Geometry: final body of the model. Coordinates: model frame, mm. A direction names the side the tool comes from. Coordinates: 2 decimals unless noted, no trailing zeros. Write each loop counter-clockwise with the first axis right and the second up, starting at its lowest first coordinate (ties: lowest second). Pieces come first, ordered by that corner, then holes.
from build123d import *

# Parameters (mm, degrees)
BOSS_EXTRUDE1_DEPTH      = 5.46
BOSS_EXTRUDE1_DEPTH_BACK = 4.7
SKETCH1_R                = 1.335
SKETCH2_W                = 6.6
SKETCH2_H                = 1.78
CUT_EXTRUDE1_DEPTH       = 29.274902299
CHAMFER1_SIZE            = 0.4
SKETCH7_R                = 1.5
CUT_EXTRUDE4_DEPTH       = 0.1
CUT_EXTRUDE5_START       = -10.06
SKETCH7_2_R              = 1.5
CUT_EXTRUDE5_DEPTH       = 0.1
SKETCH3_R                = 1.205
CUT_EXTRUDE2_DEPTH       = 2.16
SKETCH4_R                = 1.205
CUT_EXTRUDE3_DEPTH       = 2.16
BOSS_EXTRUDE2_START      = -1.52
BOSS_EXTRUDE2_DEPTH      = 0.5
LPATTERN1_COUNT          = 3
LPATTERN1_PITCH          = 2.54
LPATTERN2_COUNT          = 3
LPATTERN2_PITCH          = 2.54
BOSS_EXTRUDE3_START      = 7.6
BOSS_EXTRUDE3_DEPTH      = 1
BOSS_EXTRUDE4_START      = -8.6
BOSS_EXTRUDE4_DEPTH      = 1


with BuildPart() as part:
    # Sketch1 → Boss-Extrude1 (new, two sides: drawn at the far end of the back side and taken through both)
    with BuildSketch(Plane(origin=(0, 0, 0), x_dir=(1, 0, 0), z_dir=(0, 1, 0)).offset(-BOSS_EXTRUDE1_DEPTH_BACK)):
        Polygon((-13.335, 7.64), (13.335, 7.64), (13.335, 1.74), (7.535, -4.06), (-7.535, -4.06), (-13.335, 1.74), align=None)
        with Locations(Location((10.48, 4.75, 0), (0, 0, 270))):
            Circle(SKETCH1_R, mode=Mode.SUBTRACT)
        with Locations(Location((-10.48, 4.75, 0), (0, 0, 270))):
            Circle(SKETCH1_R, mode=Mode.SUBTRACT)
    extrude(amount=BOSS_EXTRUDE1_DEPTH + BOSS_EXTRUDE1_DEPTH_BACK)

    # Sketch2 → Cut-Extrude1 (cut, through all)
    with BuildSketch(Plane.ZY.offset(13.335)):
        with Locations((0.76, -0.89)):
            Rectangle(SKETCH2_W, SKETCH2_H)
    extrude(amount=-CUT_EXTRUDE1_DEPTH, mode=Mode.SUBTRACT)

    # Chamfer1
    chamfer1_edges = [part.edges().sort_by_distance(p)[0] for p in [
        (0, 0, 4.06),
        (0, -1.78, 4.06),
    ]]
    chamfer(chamfer1_edges, length=CHAMFER1_SIZE)

    # Sketch7 → Cut-Extrude4 (cut)
    # profile 1 of 2: a face of its own
    with BuildSketch(Plane(origin=(0, 5.46, 0), x_dir=(1, 0, 0), z_dir=(0, 1, 0))):
        with Locations(Location((0, 0, 0), (0, 0, 270))):
            Circle(SKETCH7_R)
    # profile 2 of 2: a face of its own
    with BuildSketch(Plane(origin=(0, 5.46, 0), x_dir=(1, 0, 0), z_dir=(0, 1, 0))):
        with BuildLine():
            Line((-1.5, -1.8), (1.5, -1.8))
            ThreePointArc((1.5, -1.8), (2.5, -2.8), (1.5, -3.8))
            Line((1.5, -3.8), (-1.5, -3.8))
            ThreePointArc((-1.5, -3.8), (-2.5, -2.8), (-1.5, -1.8))
        make_face()
        Polygon((-1.5, -2.8), (-0.82259388, -2.12259388), (-0.82259388, -2.482222738), (1.5, -2.482222738), (1.5, -3.117777262), (-0.82259388, -3.117777262), (-0.82259388, -3.47740612), align=None, mode=Mode.SUBTRACT)
    extrude(amount=-CUT_EXTRUDE4_DEPTH, mode=Mode.SUBTRACT)

    # Sketch7<2> → Cut-Extrude5 (cut)
    # profile 1 of 2: a face of its own
    with BuildSketch(Plane(origin=(0, 5.46, 0), x_dir=(1, 0, 0), z_dir=(0, 1, 0)).offset(CUT_EXTRUDE5_START)):
        with Locations(Location((0, 0, 0), (0, 0, 270))):
            Circle(SKETCH7_2_R)
    # profile 2 of 2: a face of its own
    with BuildSketch(Plane(origin=(0, 5.46, 0), x_dir=(1, 0, 0), z_dir=(0, 1, 0)).offset(CUT_EXTRUDE5_START)):
        with BuildLine():
            Line((-1.5, -1.8), (1.5, -1.8))
            ThreePointArc((1.5, -1.8), (2.5, -2.8), (1.5, -3.8))
            Line((1.5, -3.8), (-1.5, -3.8))
            ThreePointArc((-1.5, -3.8), (-2.5, -2.8), (-1.5, -1.8))
        make_face()
        Polygon((-1.5, -2.8), (-0.82259388, -2.12259388), (-0.82259388, -2.482222738), (1.5, -2.482222738), (1.5, -3.117777262), (-0.82259388, -3.117777262), (-0.82259388, -3.47740612), align=None, mode=Mode.SUBTRACT)
    extrude(amount=-CUT_EXTRUDE5_DEPTH, mode=Mode.SUBTRACT)

    # Sketch3 → Cut-Extrude2 (cut)
    with BuildSketch(Plane(origin=(0, 5.46, 0), x_dir=(1, 0, 0), z_dir=(0, 1, 0))):
        with Locations(Location((6.37, 4.75, 0), (0, 0, 270))):
            Circle(SKETCH3_R)
        with BuildLine():
            Line((-6.56, 5.955), (-6.18, 5.955))
            ThreePointArc((-6.18, 5.955), (-4.975, 4.75), (-6.18, 3.545))
            Line((-6.18, 3.545), (-6.56, 3.545))
            ThreePointArc((-6.56, 3.545), (-7.765, 4.75), (-6.56, 5.955))
        make_face()
    extrude(amount=-CUT_EXTRUDE2_DEPTH, mode=Mode.SUBTRACT)

    # Sketch4 → Cut-Extrude3 (cut)
    with BuildSketch(Plane.XZ.offset(4.7)):
        with Locations(Location((8.635, -1.02, 0), (0, 0, 270))):
            Circle(SKETCH4_R)
        with BuildLine():
            Line((-8.825, 0.185), (-8.445, 0.185))
            ThreePointArc((-8.445, 0.185), (-7.24, -1.02), (-8.445, -2.225))
            Line((-8.445, -2.225), (-8.825, -2.225))
            ThreePointArc((-8.825, -2.225), (-10.03, -1.02), (-8.825, 0.185))
        make_face()
    extrude(amount=-CUT_EXTRUDE3_DEPTH, mode=Mode.SUBTRACT)

    # Sketch5 → Boss-Extrude2 (add)
    with BuildSketch(Plane.XZ.offset(4.7).offset(BOSS_EXTRUDE2_START)):
        Polygon((-0.625, -7.64), (-0.625, -9.440000013), (-0.314999987, -9.749999974), (-0.314999987, -16.335000065), (0, -16.65), (0.315000013, -16.335000091), (0.315000013, -9.75), (0.625, -9.440000013), (0.625, -7.64), align=None)
    boss_extrude2 = extrude(amount=-BOSS_EXTRUDE2_DEPTH)

    # LPattern1: Boss-Extrude2 ×3
    with Locations(*[(i * LPATTERN1_PITCH, 0, 0) for i in range(1, LPATTERN1_COUNT)]):
        add(boss_extrude2)

    # LPattern2: Boss-Extrude2 ×3
    with Locations(*[(-i * LPATTERN2_PITCH, 0, 0) for i in range(1, LPATTERN2_COUNT)]):
        add(boss_extrude2)

    # Sketch6 → Boss-Extrude3 (add)
    with BuildSketch(Plane(origin=(0, 0, 0), x_dir=(0, 0, -1), z_dir=(1, 0, 0)).offset(BOSS_EXTRUDE3_START)):
        with BuildLine():
            Line((7.64, -3.18), (12.04, -3.18))
            ThreePointArc((12.04, -3.18), (12.534974747, -2.974974747), (12.74, -2.48))
            Line((12.74, -2.48), (12.74, 3.2))
            ThreePointArc((12.74, 3.2), (12.534974747, 3.694974747), (12.04, 3.9))
            Line((12.04, 3.9), (7.64, 3.9))
            Line((7.64, 3.9), (7.64, 3.4))
            Line((7.64, 3.4), (12.04, 3.4))
            ThreePointArc((12.04, 3.4), (12.181421356, 3.341421356), (12.24, 3.2))
            Line((12.24, 3.2), (12.24, -2.48))
            ThreePointArc((12.24, -2.48), (12.181421356, -2.621421356), (12.04, -2.68))
            Line((12.04, -2.68), (7.64, -2.68))
            Line((7.64, -2.68), (7.64, -3.18))
        make_face()
    extrude(amount=BOSS_EXTRUDE3_DEPTH)

    # Sketch6<2> → Boss-Extrude4 (add)
    with BuildSketch(Plane(origin=(0, 0, 0), x_dir=(0, 0, -1), z_dir=(1, 0, 0)).offset(BOSS_EXTRUDE4_START)):
        with BuildLine():
            Line((7.64, -3.18), (12.04, -3.18))
            ThreePointArc((12.04, -3.18), (12.534974747, -2.974974747), (12.74, -2.48))
            Line((12.74, -2.48), (12.74, 3.2))
            ThreePointArc((12.74, 3.2), (12.534974747, 3.694974747), (12.04, 3.9))
            Line((12.04, 3.9), (7.64, 3.9))
            Line((7.64, 3.9), (7.64, 3.4))
            Line((7.64, 3.4), (12.04, 3.4))
            ThreePointArc((12.04, 3.4), (12.181421356, 3.341421356), (12.24, 3.2))
            Line((12.24, 3.2), (12.24, -2.48))
            ThreePointArc((12.24, -2.48), (12.181421356, -2.621421356), (12.04, -2.68))
            Line((12.04, -2.68), (7.64, -2.68))
            Line((7.64, -2.68), (7.64, -3.18))
        make_face()
    extrude(amount=BOSS_EXTRUDE4_DEPTH)


solid = part.part
Item 1: Set-up query: faces 4 (the flat face through (8, -2.68, -10)), 5 (the flat face through (0, -4.6, 0)), 6 (the cylindrical face through (-7.765, 4.395, -4.724)), 7 (the flat face through (2.5, -3.18, -11.1)), 8 (the flat face through (8.6, 0.4, -12.4)). Return all of +Z, -Z, +X, -X, +Y, -Y with unobstructed straight access to the full face (end or side cutting, diameter ignored); none if empty.
Derived:
face 4: +X, -X
face 5: -Y
face 6: +Y
face 7: -Z, +X, -X, -Y
face 8: -Z, +X, +Y, -Y
Item 2: Section B-B, the plane z = -4.75. Output: boundary loops of the cut face in (x, y) (3 decimals).
Derived:
outline: (-13.335, -4.7) - (-11.815, -4.7) - (-11.815, 5.46) - (-13.335, 5.46) - close; (-9.145, -4.7) - (9.145, -4.7) - (9.145, 5.46) - (7.575, 5.46) - (7.575, 3.3) - (5.165, 3.3) - (5.165, 5.46) - (-4.975, 5.46) - (-4.975, 3.3) - (-7.765, 3.3) - (-7.765, 5.46) - (-9.145, 5.46) - close; (11.815, -4.7) - (13.335, -4.7) - (13.335, 5.46) - (11.815, 5.46) - close
Item 3: Section D-D, the plane z = -1.02. Output: boundary loops of the cut face in (x, y) (3 decimals).
Derived:
outline: (-12.615, -4.7) - (-10.03, -4.7) - (-10.03, -2.54) - (-7.24, -2.54) - (-7.24, -4.7) - (-1.1, -4.7) - (-1.1, -4.6) - (1.1, -4.6) - (1.1, -4.7) - (7.43, -4.7) - (7.43, -2.54) - (9.84, -2.54) - (9.84, -4.7) - (12.615, -4.7) - (12.615, -1.78) - (-12.615, -1.78) - close; (-12.615, 0) - (12.615, 0) - (12.615, 5.46) - (1.1, 5.46) - (1.1, 5.36) - (-1.1, 5.36) - (-1.1, 5.46) - (-12.615, 5.46) - close
Item 4: Material intervals for probe 1 along X at (y, z) = (3, -4.75) (3 decimals); probe 2 along X at (y, z) = (-3.65, -1.02) (3 decimals); probe 3 along Y at (x, z) = (-2.25, -1.25), sorted ascending.
Derived:
probe 1: x = -13.335 to -11.815, -9.145 to 9.145, 11.815 to 13.335
probe 2: x = -12.615 to -10.03, -7.24 to 7.43, 9.84 to 12.615
probe 3: y = -4.7 to -1.78, 0 to 5.46
Item 5: Section C-C, the plane x = 6.37. Output: boundary loops of the cut face in (y, z) (3 decimals), plus the area to 3 significant figures.
Derived:
outline: (-4.7, -7.64) - (5.46, -7.64) - (5.46, -5.955) - (3.3, -5.955) - (3.3, -3.545) - (5.46, -3.545) - (5.46, 4.06) - (0.4, 4.06) - (0, 3.66) - (0, -2.54) - (-1.78, -2.54) - (-1.78, 3.66) - (-2.18, 4.06) - (-4.7, 4.06) - close
area: 102 mm2
Item 6: Pull-direction query (Z, two-part tool) for faces 1 (the flat face through (0, -1.78, 1)), 2 (the flat face through (-8, 0, -12.74)), 3 (the flat face through (-6, 3.3, -5)); classes: released by +Z, released by -Z, zero draft, split by the parting line, or undercut.
Derived:
face 1: zero draft
face 2: released by -Z
face 3: undercut
Item 7: Pin query (flat end, axial travel): pin 1 (0.6 mm diameter, centred on y = -3, z = -8.5, fed in from +X); pin 2 (1.1 mm diameter, centred on x = -8, z = -11, fed in from +Y); pin 3 (5 mm diameter, centred on x = -2, y = 1, fed in from -Z). Return the tip coordinate at first contact, or that it passes through.
Derived:
pin 1: stops at x = 8.6
pin 2: stops at y = 3.9
pin 3: stops at z = -7.64
Item 8: Section A-A, the plane y = -1.25. Output: boundary loops of the cut face in (x, z) (3 decimals), plus the area to 3 significant figures.
Derived:
outline: (-13.335, -7.64) - (13.335, -7.64) - (13.335, -2.54) - (-13.335, -2.54) - close; (-8.6, -12.74) - (-7.6, -12.74) - (-7.6, -12.24) - (-8.6, -12.24) - close; (7.6, -12.74) - (8.6, -12.74) - (8.6, -12.24) - (7.6, -12.24) - close; hole circle Ø2.67 at (-10.48, -4.75); hole circle Ø2.67 at (10.48, -4.75)
area: 126 mm2
